from build123d import *

# Parameters (mm, degrees)
SKETCH1_W           = 36.7
SKETCH1_H           = 34.9
SKETCH1_W_2         = 34.7
SKETCH1_H_2         = 32.9
BOSS_EXTRUDE1_DEPTH = 8
SKETCH2_W           = 36.7
SKETCH2_H           = 34.9
BOSS_EXTRUDE2_DEPTH = 4.2
SKETCH3_W           = 4.9
SKETCH3_H           = 1
CUT_EXTRUDE1_DEPTH  = 4.5
SKETCH4_W           = 9.6
SKETCH4_H           = 1
CUT_EXTRUDE2_DEPTH  = 8
SKETCH5_W           = 34.7
SKETCH5_H           = 1.5
BOSS_EXTRUDE3_DEPTH = 1.6
SKETCH6_W           = 34.7
SKETCH6_H           = 31.4
CUT_EXTRUDE3_DEPTH  = 2


with BuildPart() as part:
    # Sketch1 → Boss-Extrude1 (new body)
    with BuildSketch(Plane.XY):
        with Locations((18.35, 17.45)):
            Rectangle(SKETCH1_W, SKETCH1_H)
        with Locations((18.35, 17.45)):
            Rectangle(SKETCH1_W_2, SKETCH1_H_2, mode=Mode.SUBTRACT)
    extrude(amount=BOSS_EXTRUDE1_DEPTH)

    # Sketch2 → Boss-Extrude2 (add)
    with BuildSketch(Plane(origin=(0, 0, 0), x_dir=(-1, 0, 0), z_dir=(0, 0, -1))):
        with Locations((-18.35, 17.45)):
            Rectangle(SKETCH2_W, SKETCH2_H)
    extrude(amount=BOSS_EXTRUDE2_DEPTH)

    # Sketch3 → Cut-Extrude1 (cut)
    with BuildSketch(Plane.XY.offset(8)):
        with Locations((28.25, 0.5)):
            Rectangle(SKETCH3_W, SKETCH3_H)
    extrude(amount=-CUT_EXTRUDE1_DEPTH, mode=Mode.SUBTRACT)

    # Sketch4 → Cut-Extrude2 (cut)
    with BuildSketch(Plane.XY.offset(8)):
        with Locations((17.7, 0.5)):
            Rectangle(SKETCH4_W, SKETCH4_H)
    extrude(amount=-CUT_EXTRUDE2_DEPTH, mode=Mode.SUBTRACT)

    # Sketch5 → Boss-Extrude3 (add)
    with BuildSketch(Plane.XY):
        with Locations((18.35, 33.15)):
            Rectangle(SKETCH5_W, SKETCH5_H)
    extrude(amount=BOSS_EXTRUDE3_DEPTH)

    # Sketch6 → Cut-Extrude3 (cut)
    with BuildSketch(Plane.XY):
        with Locations((18.35, 16.7)):
            Rectangle(SKETCH6_W, SKETCH6_H)
    extrude(amount=-CUT_EXTRUDE3_DEPTH, mode=Mode.SUBTRACT)


solid = part.part
Could you check a few things on this model? Use its own coordinates, in mm. A direction names the side the tool comes from. Give positions to 0.01 mm unless a question says otherwise; leave off trailing zeros. Loops run counter-clockwise (first coordinate to the right, second up) from the corner with the lowest first, then second, coordinate; pieces in that order, holes last. Notation, with made-up numbers: M 23,57.5 L 38,57.5 A24 ccw 38,75.5 Z; hole C 46.5,19.25 d1. An arc over 180 degrees is marked long. Answer as a JSON object with one key per item and string values.
Q1. Suppose I cut it at C-C, the plane z = -1. List the corners of the cut face in (x, y) for me, plus the area to 3 significant figures.
Values found:
{"outline": "M 0,0 L 36.7,0 L 36.7,34.9 L 0,34.9 Z; hole M 1,1 L 35.7,1 L 35.7,32.4 L 1,32.4 Z", "area": "191 mm²"}
Q2. Suppose I cut it at B-B, the plane x = 11.5. List the corners of the cut face in (y, z) for me, plus the area to 3 significant figures.
Values found:
{"outline": "M 0,-4.2 L 34.9,-4.2 L 34.9,8 L 33.9,8 L 33.9,1.6 L 32.4,1.6 L 32.4,-2 L 1,-2 L 1,8 L 0,8 Z", "area": "102 mm²"}
Q3. For P1, Ø1.6, axis at x = 12.5, y = 33, coming from the +Z side; P2, Ø9.5, axis at x = 23, y = 22.5, coming from the +Z side; P3, Ø0.8, axis at x = 28, y = 0.5, coming from the +Z side, each with a flat end and sliding along its axis, tell me the tip position at first contact or that it passes through.
Values found:
{"P1": "stops at z = 1.6", "P2": "stops at z = -2", "P3": "stops at z = 3.5"}
Q4. Suppose I cut it at A-A, the plane z = 7.25. List the corners of the cut face in (x, y) for me, plus the area to 3 significant figures.
Values found:
{"outline": "M 0,0 L 12.9,0 L 12.9,1 L 1,1 L 1,33.9 L 35.7,33.9 L 35.7,1 L 30.7,1 L 30.7,0 L 36.7,0 L 36.7,34.9 L 0,34.9 Z; M 22.5,0 L 25.8,0 L 25.8,1 L 22.5,1 Z", "area": "125 mm²"}
Q5. If I drill on probe 1 along Y at (x, z) = (31, 4); probe 2 along Y at (x, z) = (24, -1.5); probe 3 along X at (y, z) = (2.5, 1.5), over which ranges is the centre line in solid material (lowest first)? Write a range as [from, to].
Values found:
{"probe 1": "y = [0, 1], [33.9, 34.9]", "probe 2": "y = [0, 1], [32.4, 34.9]", "probe 3": "x = [0, 1], [35.7, 36.7]"}
Q6. Suppose I cut it at D-D, the plane y = 33. List the corners of the cut face in (x, z) for me, plus the area to 3 significant figures.
Values found:
{"outline": "M 0,-4.2 L 36.7,-4.2 L 36.7,8 L 35.7,8 L 35.7,1.6 L 1,1.6 L 1,8 L 0,8 Z", "area": "226 mm²"}
Q7. For faces 5 (the flat face through (16.9, 34.3, 8)), 6 (the flat face through (18, 17, -2)), 7 (the flat face through (22.5, 0.5, 4.1)), which set-ups out of +Z, -Z, +X, -X, +Y, -Y let a thin tool reach every point of the face, with its end or its side?
Values found:
{"face 5": "+Z, +X, -X, +Y, -Y", "face 6": "+Z", "face 7": "+Z, -Y"}
Q8. If we mould it in two halves opening along Y, with no side actions, what happens to faces 1 (the flat face through (19, 0, -1)), 2 (the flat face through (28.2, 0.5, 3.5)), 3 (the flat face through (1, 17, 3)), 4 (the flat face through (35.7, 17, 3))? For each: pulls with the +Y half, pulls with the -Y half, needs draft (parallel to the pull), parting line crosses it, or undercut.
Values found:
{"face 1": "pulls with the -Y half", "face 2": "needs draft", "face 3": "undercut", "face 4": "undercut"}
